The listing builds one solid part. Answer for the finished solid, in the listing's coordinates (mm). Give positions to 0.01 mm unless a question says otherwise; leave off trailing zeros. Write each loop counter-clockwise with the first axis right and the second up, starting at its lowest first coordinate (ties: lowest second). Pieces come first, ordered by that corner, then holes. Notation, with made-up numbers: (12.25, -36.75) - (42.25, -36.75) arc R24 cw to (42.25, -11.75) - close; hole circle Ø4 at (-39, -3.75). An arc over 180 degrees is marked (long way). Return JSON: item names as keys, results as strings.
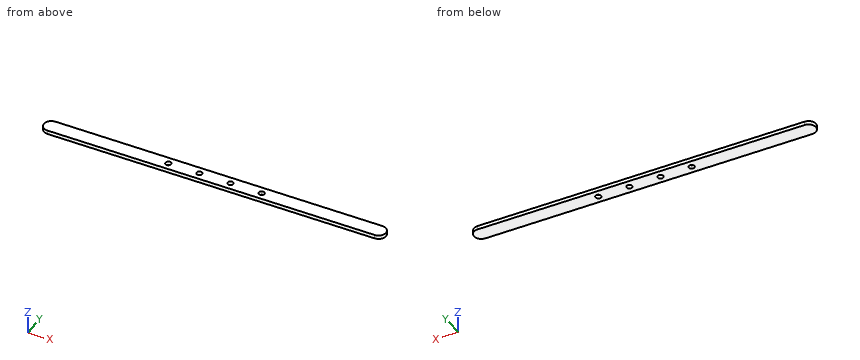
from build123d import *

# Parameters (mm, degrees)
SKETCH1_W           = 550
SKETCH1_H           = 24
SKETCH1_R           = 4.5
BOSS_EXTRUDE1_DEPTH = 6
FILLET2_R           = 12


with BuildPart() as part:
    # Sketch1 → Boss-Extrude1 (new body)
    with BuildSketch(Plane.XY):
        Rectangle(SKETCH1_W, SKETCH1_H)
        with Locations((75, 0)):
            Circle(SKETCH1_R, mode=Mode.SUBTRACT)
        with Locations((25, 0)):
            Circle(SKETCH1_R, mode=Mode.SUBTRACT)
        with Locations((-25, 0)):
            Circle(SKETCH1_R, mode=Mode.SUBTRACT)
        with Locations((-75, 0)):
            Circle(SKETCH1_R, mode=Mode.SUBTRACT)
    extrude(amount=BOSS_EXTRUDE1_DEPTH)

    # Fillet2
    fillet2_edges = [part.edges().sort_by_distance(p)[0] for p in [
        (-275, -12, 3),
        (-275, 12, 3),
        (275, 12, 3),
        (275, -12, 3),
    ]]
    fillet(fillet2_edges, radius=FILLET2_R - 0.0001)  # a hair under: the kernel refuses the full size


solid = part.part
Item 1: Consider L1, parallel to Y at x = -25, z = 4.3; L2, parallel to X at y = -1.5, z = 0.75; L3, parallel to X at y = 7, z = 1.9. Determine where each line is inside the solid, lowest interval first.
Answer below:
{"L1": "y = -12 to -4.5, 4.5 to 12", "L2": "x = -274.91 to -79.24, -70.76 to -29.24, -20.76 to 20.76, 29.24 to 70.76, 79.24 to 274.91", "L3": "x = -272.75 to 272.75"}
Item 2: A cutting plane is placed at B-B on x = 25. Determine the outline of the cut face in (y, z).
Answer below:
{"outline": "(-12, 0) - (-4.5, 0) - (-4.5, 6) - (-12, 6) - close; (4.5, 0) - (12, 0) - (12, 6) - (4.5, 6) - close"}
Item 3: Flat-ended cylindrical pins translate along their axes: P1, Ø7, axis at x = -25, y = 0, coming from the -Z side; P2, Ø1, axis at y = -4.5, z = 3.5, coming from the +X side; P3, Ø1.5, axis at y = 4.5, z = 1.5, coming from the -X side. Find the tip coordinate at first contact, or state that the pin passes through.
Answer below:
{"P1": "passes through", "P2": "stops at x = 274.31", "P3": "stops at x = -274.4"}
Item 4: A cutting plane is placed at A-A on z = 2.4. Give the number of separate pieces and of enclosed holes in the cut face, then the cut area to 3 significant figures.
Answer below:
{"separate pieces": "1", "enclosed holes": "4", "area": "12,800 mm²"}
